For this review, take the finished solid that the model builds, in its own axes (mm). A direction names the side the tool comes from. Coordinates: 2 decimals unless noted, no trailing zeros. Order: outer loops, then holes, each group sorted by start corner. A loop starts at its lowest first (then second) coordinate and runs counter-clockwise, first axis right, second up. Notation, with made-up numbers: (-10, 44.5) -> (19, 44.5) arc R21 ccw to (19, 61.5) -> close; hole circle Ø1 at (-0.5, -17). An arc over 180 degrees is marked (long way). Write item = value, one per line. Start each with the question number.
1) Consider section B-B on y = 4.5. Give the boundary of the cut face in (x, z), and give its area (3 significant figures).
2) Wall thickness on probe 1 along X at (y, z) = (8.5, 6.5); probe 2 along Y at (x, z) = (-20.5, 3.5); probe 3 along Y at (x, z) = (-5, -6.5): over which ranges is each line inside the solid? List them lowest first. Write a range as [from, to].
3) Consider section C-C on z = 11. Give the boundary of the cut face in (x, y).
4) Consider section D-D on y = 12.5. Give the boundary of the cut face in (x, z).
5) Insertion check: pin 1 Ø6 at (x, z) = (-15, -8.5) entering from -Y; pin 2 Ø4 at (x, z) = (-33, -8) entering from -Y; pin 3 Ø1 at (y, z) = (-2.5, 12) entering from -X; pin 4 Ø1 at (x, z) = (-34, -9) entering from +Y. Each pin has a flat end and moves straight along its axis. Give the tip position at first contact, or say it passes through.
6) Machinability: for faces 1 (the face through (-19.72, -5.361, -5.245)), 2 (the face through (0, -4, 7)), 3 (the face through (-19.72, 5.361, 5.245)), 4 (the face through (-19.72, -5.361, 5.245)), which of the approach directions +Z, -Z, +X, -X, +Y, -Y give a long, thin tool a straight path to every point of the face, cutting with its end or side? Answer none if there is none.
from build123d import *

# Parameters (mm, degrees)
F2_DEPTH = 5
F1_W     = 40
F1_H     = 15
F3_DEPTH = 7.5
F4_R     = 7.49999


# Not quite as in the source:
# - a fillet or chamfer is up to 0.001 mm smaller than in the source, because OpenCascade refuses the exact size


with BuildPart() as f2:
    # F0 (on Right) → F2 (new body)
    with BuildSketch(Plane.YZ):
        Polygon((15.3302561211, -6.35), (15.3302561211, 6.35), (6.35, 15.3302561211), (-6.35, 15.3302561211), (-15.3302561211, 6.35), (-15.3302561211, -6.35), (-6.35, -15.3302561211), (6.35, -15.3302561211), align=None)
    extrude(amount=F2_DEPTH)

    # F1 (on Top) → F3 (join, symmetric)
    with BuildSketch(Plane.XY):
        with Locations((-20, 0)):
            Rectangle(F1_W, F1_H)
    extrude(amount=F3_DEPTH, both=True)

    # F4 (radius 7.5 in the source; OpenCascade refuses exactly that, so slightly less here)
    f4_edges = [f2.edges().sort_by_distance(p)[0] for p in [
        (-20, 7.5, 7.5),
        (-20, 7.5, -7.5),
        (-20, -7.5, -7.5),
        (-20, -7.5, 7.5),
    ]]
    fillet(f4_edges, radius=F4_R)


solid = f2.part
Answer sheet:
q1.outline = (-40, -6) -> (0, -6) -> (0, -15.33) -> (5, -15.33) -> (5, 15.33) -> (0, 15.33) -> (0, 6) -> (-40, 6) -> close
q1.area = 633 mm2
q2.probe_1 = [0, 5]
q2.probe_2 = [-6.63, 6.63]
q2.probe_3 = [-3.74, 3.74]
q3.outline = (0, -10.68) -> (5, -10.68) -> (5, 10.68) -> (0, 10.68) -> close
q4.outline = (0, -9.18) -> (5, -9.18) -> (5, 9.18) -> (0, 9.18) -> close
q5.pin_1 = -5.1
q5.pin_2 = -4.5
q5.pin_3 = 0
q5.pin_4 = through
q6.face_1 = -Z, -X, -Y
q6.face_2 = +Z, -X, -Y
q6.face_3 = +Z, -X, +Y
q6.face_4 = +Z, -X, -Y
